from build123d import *

# Parameters (mm, degrees)
SALIENTE_EXTRUIR1_DEPTH = 394
CROQUIS2_R              = 3
CROQUIS2_R_2            = 15
CORTAR_EXTRUIR1_DEPTH   = 425.673777624
CROQUIS4_R              = 8
CORTAR_EXTRUIR3_DEPTH   = 426.218662567
CROQUIS5_R              = 7.5
SALIENTE_EXTRUIR2_DEPTH = 78
CROQUIS6_R              = 6
SALIENTE_EXTRUIR3_DEPTH = 120
CORTAR_EXTRUIR4_DEPTH   = 439.873456699


with BuildPart() as part:
    # Croquis1 → Saliente-Extruir1 (new body)
    with BuildSketch(Plane.XY):
        with BuildLine():
            Line((96.164660939, 24.571471574), (100.927160939, 24.571471574))
            Line((100.927160939, 24.571471574), (100.927160939, 136.808971574))
            ThreePointArc((100.927160939, 136.808971574), (96.603324796, 147.247635431), (86.164660939, 151.571471574))
            Line((86.164660939, 151.571471574), (49.927160939, 151.571471574))
            Line((49.927160939, 151.571471574), (49.927160939, 146.808971574))
            Line((49.927160939, 146.808971574), (86.164660939, 146.808971574))
            ThreePointArc((86.164660939, 146.808971574), (93.235728751, 143.880039386), (96.164660939, 136.808971574))
            Line((96.164660939, 136.808971574), (96.164660939, 24.571471574))
        make_face()
    extrude(amount=-SALIENTE_EXTRUIR1_DEPTH)

    # Croquis2 → Cortar-Extruir1 (cut, through all)
    with BuildSketch(Plane.ZY.offset(-96.164660939)):
        with Locations(Location((-40, 36.973884985, 0), (0, 0, 180))):
            Circle(CROQUIS2_R)
        with Locations(Location((-12.402413411, 64.571471574, 0), (0, 0, 180))):
            Circle(CROQUIS2_R)
        with Locations(Location((-67.597586589, 64.571471574, 0), (0, 0, 180))):
            Circle(CROQUIS2_R)
        with Locations(Location((-40, 92.169058163, 0), (0, 0, 180))):
            Circle(CROQUIS2_R)
        with Locations(Location((-40, 64.571471574, 0), (0, 0, 180))):
            Circle(CROQUIS2_R_2)
        with Locations(Location((-326.402413411, 94.571471574, 0), (0, 0, 180))):
            Circle(CROQUIS2_R)
        with Locations(Location((-354, 66.973884985, 0), (0, 0, 180))):
            Circle(CROQUIS2_R)
        with Locations(Location((-354, 94.571471574, 0), (0, 0, 180))):
            Circle(CROQUIS2_R_2)
        with Locations(Location((-381.597586589, 94.571471574, 0), (0, 0, 180))):
            Circle(CROQUIS2_R)
        with Locations(Location((-354, 122.169058163, 0), (0, 0, 180))):
            Circle(CROQUIS2_R)
    extrude(amount=-CORTAR_EXTRUIR1_DEPTH, mode=Mode.SUBTRACT)

    # Croquis4 → Cortar-Extruir3 (cut, through all)
    with BuildSketch(Plane(origin=(100.927160939, 0, 0), x_dir=(0, 0, -1), z_dir=(1, 0, 0))):
        with Locations(Location((30, 114.571471574, 0), (0, 0, 90))):
            Circle(CROQUIS4_R)
    extrude(amount=-CORTAR_EXTRUIR3_DEPTH, mode=Mode.SUBTRACT)

    # Croquis5 → Saliente-Extruir2 (add)
    with BuildSketch(Plane(origin=(100.927160939, 0, 0), x_dir=(0, 0, -1), z_dir=(1, 0, 0))):
        with Locations(Location((84, 96.571471574, 0), (0, 0, 90))):
            Circle(CROQUIS5_R)
    extrude(amount=SALIENTE_EXTRUIR2_DEPTH)

    # Croquis6 → Saliente-Extruir3 (add)
    with BuildSketch(Plane(origin=(100.927160939, 0, 0), x_dir=(0, 0, -1), z_dir=(1, 0, 0))):
        with Locations(Location((316, 129.571471574, 0), (0, 0, 90))):
            Circle(CROQUIS6_R)
    extrude(amount=SALIENTE_EXTRUIR3_DEPTH)

    # Croquis7 → Cortar-Extruir4 (cut, through all)
    with BuildSketch(Plane(origin=(100.927160939, 0, 0), x_dir=(0, 0, -1), z_dir=(1, 0, 0))):
        with BuildLine():
            Line((47, 133.571471574), (201, 133.571471574))
            ThreePointArc((201, 133.571471574), (206, 128.571471574), (201, 123.571471574))
            Line((201, 123.571471574), (47, 123.571471574))
            ThreePointArc((47, 123.571471574), (42, 128.571471574), (47, 133.571471574))
        make_face()
    extrude(amount=-CORTAR_EXTRUIR4_DEPTH, mode=Mode.SUBTRACT)


solid = part.part
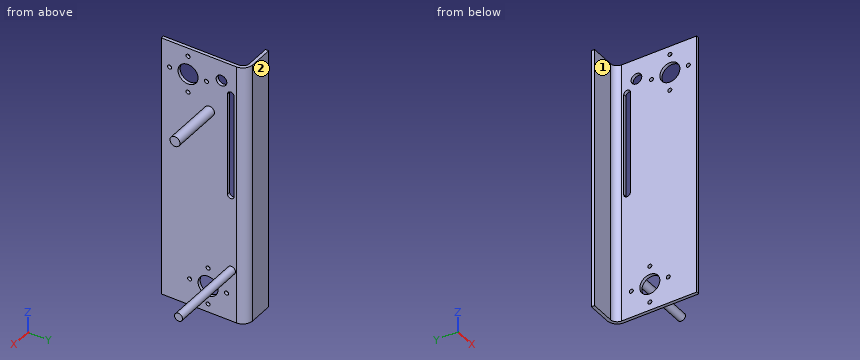
Geometry check sheet. Reference: the model listing, model coordinates, mm. Face numbers are marked on the shaded views. A direction names the side the tool comes from. Coordinates: 2 decimals unless noted, no trailing zeros. Order: outer loops, then holes, each group sorted by start corner. A loop starts at its lowest first (then second) coordinate and runs counter-clockwise, first axis right, second up. Notation, with made-up numbers: (18.5, 71.5) -> (39.5, 71.5) arc R24 cw to (39.5, 110.5) -> close; hole circle Ø7 at (37.25, 22.5). An arc over 180 degrees is marked (long way). Use a Markdown table: item, result. Add a question column.
1. Set-up check for the marked faces 1 and 2: record each of +Z, -Z, +X, -X, +Y, -Y from which the full face is reachable in a straight line by a thin tool's end or side.
2. Material ranges on L1, parallel to X at y = 55.5, z = -356; L2, parallel to Y at x = 98.75, z = -354; L3, parallel to Y at x = 97.2, z = -40, recorded low to high.
3. Cross-section at B-B (z = -292.5). Enter the section's corners in (x, y) (1 decimal), and give its area (3 significant figures).
4. Cross-section at C-C (z = -30). Enter the section's corners in (x, y) (1 decimal), and give its area (3 significant figures).
5. Cross-section at A-A (z = -183). Enter the section's corners in (x, y) (1 decimal), and give its area (3 significant figures).
6. Go/stop test with flat-tipped pins: pin 1 Ø5.5 at (y, z) = (94.57, -381.6) entering from +X; pin 2 Ø10 at (y, z) = (48.5, -52.5) entering from -X; pin 3 Ø4 at (y, z) = (41, -307) entering from +X; pin 4 Ø12 at (y, z) = (99.5, -86) entering from +X. Record where each tip stops, or that it passes through.
Filled sheet:
| question | item | result |
|---|---|---|
| 1 | face 1 | +Z, -Z, -X, -Y |
| 1 | face 2 | +Z, -Z, +X, -X, +Y |
| 2 | L1 | 96.16 to 100.93 |
| 2 | L2 | 24.57 to 63.97, 69.97 to 79.57, 109.57 to 119.17, 125.17 to 144.53 |
| 2 | L3 | 24.57 to 33.97, 39.97 to 49.57, 79.57 to 89.17, 95.17 to 146.61 |
| 3 | outline | (49.9, 146.8) -> (86.2, 146.8) arc R10 cw to (96.2, 136.8) -> (96.2, 24.6) -> (100.9, 24.6) -> (100.9, 136.8) arc R14.8 ccw to (86.2, 151.6) -> (49.9, 151.6) -> close |
| 3 | area | 800 mm2 |
| 4 | outline | (49.9, 146.8) -> (86.2, 146.8) arc R10 cw to (96.2, 136.8) -> (96.2, 122.6) -> (100.9, 122.6) -> (100.9, 136.8) arc R14.8 ccw to (86.2, 151.6) -> (49.9, 151.6) -> close; (96.2, 24.6) -> (100.9, 24.6) -> (100.9, 53.4) -> (96.2, 53.4) -> close; (96.2, 75.8) -> (100.9, 75.8) -> (100.9, 106.6) -> (96.2, 106.6) -> close |
| 4 | area | 617 mm2 |
| 5 | outline | (49.9, 146.8) -> (86.2, 146.8) arc R10 cw to (96.2, 136.8) -> (96.2, 133.6) -> (100.9, 133.6) -> (100.9, 136.8) arc R14.8 ccw to (86.2, 151.6) -> (49.9, 151.6) -> close; (96.2, 24.6) -> (100.9, 24.6) -> (100.9, 123.6) -> (96.2, 123.6) -> close |
| 5 | area | 752 mm2 |
| 6 | pin 1 | through |
| 6 | pin 2 | x = 96.16 |
| 6 | pin 3 | x = 100.93 |
| 6 | pin 4 | x = 178.93 |
